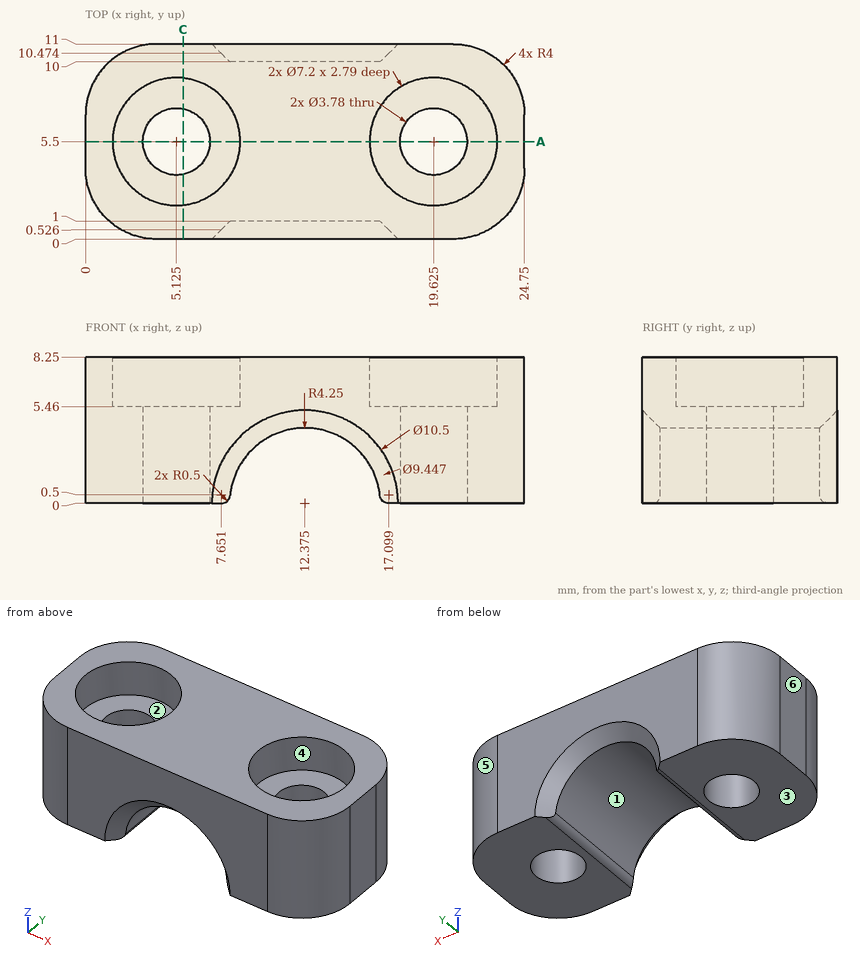
Source: three-view drawing plus pictorial views. Frame: mm from the lowest corner of the part. A direction names the side the tool comes from. Round coordinates to 2 decimals unless told otherwise and drop trailing zeros. Order: outer loops, then holes, each group sorted by start corner. A loop starts at its lowest first (then second) coordinate and runs counter-clockwise, first axis right, second up. Notation, with made-up numbers: (27.5, 88) - (57.5, 88) arc R22 ccw to (57.5, 121) - close; hole circle Ø4 at (16.5, 74.5). An arc over 180 degrees is marked (long way). Answer in a Markdown table with one row per item.
Item 1: Mould query, pull axis X, two halves, no side actions, for the marked faces 3, 4, 5 and 6. Classes: released by +X, released by -X, zero draft, split by the parting line, or undercut.
Model answer:
| item | result |
|---|---|
| face 3 | zero draft |
| face 4 | undercut |
| face 5 | released by +X |
| face 6 | released by -X |
Item 2: Section query C-C (x = 5.5). Return the cut outline in (y, z).
Model answer:
| item | result |
|---|---|
| outline | (0, 0) - (3.65, 0) - (3.65, 5.46) - (1.92, 5.46) - (1.92, 8.25) - (0, 8.25) - close; (7.35, 0) - (11, 0) - (11, 8.25) - (9.08, 8.25) - (9.08, 5.46) - (7.35, 5.46) - close |
Item 3: Section query A-A (y = 5.5). Give the number of separate pieces and of enclosed holes in the cut face.
Model answer:
| item | result |
|---|---|
| separate pieces | 3 |
| enclosed holes | 0 |
Item 4: Reachability of the marked faces 1 and 2 from +Z, -Z, +X, -X, +Y, -Y: full face, straight path, thin tool, end or side. Return the list, or none.
Model answer:
| item | result |
|---|---|
| face 1 | -Z, +Y, -Y |
| face 2 | +Z |
Item 5: Pin query (flat end, axial travel): pin 1 (2 mm diameter, centred on x = 19.5, y = 7, fed in from +Z); pin 2 (3 mm diameter, centred on x = 5.125, y = 5.5, fed in from -Z). Return the tip coordinate at first contact, or that it passes through.
Model answer:
| item | result |
|---|---|
| pin 1 | stops at z = 5.46 |
| pin 2 | passes through |
Item 6: Line query: line 1 (Z direction, x = 7, y = 7.25); line 2 (X direction, y = 5.25, z = 7.75); line 3 (X direction, y = 2, z = 3.5) (1 decimal). Output: solid intervals per line, ascending.
Model answer:
| item | result |
|---|---|
| line 1 | z = 0 to 5.46 |
| line 2 | x = 0 to 1.53, 8.72 to 16.03, 23.22 to 24.75 |
| line 3 | x = 0.5 to 10, 14.8 to 24.2 |
